The listing builds one solid part. Answer for the finished solid, in the listing's coordinates (mm). A direction names the side the tool comes from. Round coordinates to 2 decimals unless told otherwise and drop trailing zeros. Write each loop counter-clockwise with the first axis right and the second up, starting at its lowest first coordinate (ties: lowest second). Pieces come first, ordered by that corner, then holes.
Item 1: Find section A-A on z = 23. Give the vertices of the cut face in (x, y), then the cut area to 4 significant figures.
Item 2: Find section D-D on z = 9. Give the number of separate pieces and of enclosed holes in the cut face, then the cut area to 3 significant figures.
Item 3: For a pull along Y with two mould halves and no side action, classify faces 3 (the face through (-1, 34.5, 20)), 4 (the face through (-40.337, -31.317, 20.28)), 5 (the face through (-33.61, -21.49, 7.53)), 6 (the face through (-44.5, 0, 20)) as +Y half, -Y half, draft (parallel to the pull), parting line (faces both ways), or undercut.
Item 4: Each of these flat-tipped pins is pushed along its axis until it touches: pin 1 (18 mm diameter, centred on x = -4.5, y = 6.5, fed in from +Z); pin 2 (1.8 mm diameter, centred on x = -33.5, y = -21, fed in from +Z). Where does it stop, or does it pass through?
Item 5: Find section C-C on y = -22.5. Give the vertices of the cut face in (x, z).
Item 6: Find the intervals of material crossed by probe 1 along X at (y, z) = (-3, 37); probe 2 along Y at (x, z) = (15, 19.5); probe 3 along Y at (x, z) = (-32.5, 6.2), in increasing order.
Item 7: Find section B-B on x = 19.5. Give the vertices of the cut face in (y, z), then the cut area to 3 significant figures.
Item 8: A tool of negligible diameter and unlimited length cuts with its end or side. For faces 1 (the face through (-1, -30, 23)), 2 (the face through (0, -31, 40)), from which of +Z, -Z, +X, -X, +Y, -Y can it reach the whole face along a straight path? Write none if from no direction.
```python
from build123d import *

# Parameters (mm, degrees)
SKETCH_W        = 89
SKETCH_H        = 69
PAD_DEPTH       = 40
SKETCH001_W     = 80
SKETCH001_H     = 60
SKETCH001_R     = 3
SKETCH001_R_2   = 1.5
POCKET_DEPTH    = 35
SKETCH002_R     = 1.5
POCKET001_DEPTH = 40.001
SKETCH003_W     = 76.892074
SKETCH003_H     = 56.42009
POCKET002_DEPTH = 30
FILLET_R        = 3


with BuildPart() as part:
    # Sketch → Pad (new body)
    with BuildSketch(Plane.XY):
        Rectangle(SKETCH_W, SKETCH_H)
    extrude(amount=PAD_DEPTH)

    # Sketch001 (on DatumPlane) → Pocket (cut)
    with BuildSketch(Plane.XY.offset(40)):
        Rectangle(SKETCH001_W, SKETCH001_H)
        with Locations((-32.5, 22.5)):
            Circle(SKETCH001_R, mode=Mode.SUBTRACT)
        with Locations((32.5, 22.5)):
            Circle(SKETCH001_R, mode=Mode.SUBTRACT)
        with Locations((32.5, -22.5)):
            Circle(SKETCH001_R, mode=Mode.SUBTRACT)
        with Locations((-32.5, -22.5)):
            Circle(SKETCH001_R, mode=Mode.SUBTRACT)
        with Locations((-32.5, 22.5)):
            Circle(SKETCH001_R_2)
        with Locations((32.5, 22.5)):
            Circle(SKETCH001_R_2)
        with Locations((32.5, -22.5)):
            Circle(SKETCH001_R_2)
        with Locations((-32.5, -22.5)):
            Circle(SKETCH001_R_2)
    extrude(amount=-POCKET_DEPTH, mode=Mode.SUBTRACT)

    # Sketch002 (on DatumPlane) → Pocket001 (cut, through all)
    with BuildSketch(Plane.XY.offset(40)):
        with Locations((41.767767, 31.767767)):
            Circle(SKETCH002_R)
        with Locations((41.767767, -31.767767)):
            Circle(SKETCH002_R)
        with Locations((-41.767767, -31.767767)):
            Circle(SKETCH002_R)
        with Locations((-41.767767, 31.767767)):
            Circle(SKETCH002_R)
    extrude(amount=-POCKET001_DEPTH, mode=Mode.SUBTRACT)

    # Sketch003 (on DatumPlane) → Pocket002 (cut)
    with BuildSketch(Plane.XY.offset(40)):
        Rectangle(SKETCH003_W, SKETCH003_H)
    extrude(amount=-POCKET002_DEPTH, mode=Mode.SUBTRACT)

    # Fillet
    fillet_edges = [part.edges().sort_by_distance(p)[0] for p in [
        (-44.5, -34.5, 20),
        (44.5, -34.5, 20),
        (44.5, 34.5, 20),
        (-44.5, 34.5, 20),
    ]]
    fillet(fillet_edges, radius=FILLET_R)


solid = part.part
```
Check values:
1. outline: (-44.5, -31.5) arc R3 ccw to (-41.5, -34.5) - (41.5, -34.5) arc R3 ccw to (44.5, -31.5) - (44.5, 31.5) arc R3 ccw to (41.5, 34.5) - (-41.5, 34.5) arc R3 ccw to (-44.5, 31.5) - close; hole circle Ø3 at (-41.77, -31.77); hole circle Ø3 at (-41.77, 31.77); hole (-40, -30) - (40, -30) - (40, 30) - (-40, 30) - close; hole circle Ø3 at (41.77, -31.77); hole circle Ø3 at (41.77, 31.77)
1. area: 1,305 mm2
2. separate pieces: 5
2. enclosed holes: 9
2. area: 1,390 mm2
3. face 3: +Y half
3. face 4: undercut
3. face 5: undercut
3. face 6: draft
4. pin 1: stops at z = 5
4. pin 2: stops at z = 10
5. outline: (-44.5, 0) - (44.5, 0) - (44.5, 40) - (40, 40) - (40, 5) - (35.5, 5) - (35.5, 10) - (34, 10) - (34, 5) - (31, 5) - (31, 10) - (29.5, 10) - (29.5, 5) - (-29.5, 5) - (-29.5, 10) - (-31, 10) - (-31, 5) - (-34, 5) - (-34, 10) - (-35.5, 10) - (-35.5, 5) - (-40, 5) - (-40, 40) - (-44.5, 40) - close
6. probe 1: x = -44.5 to -40, 40 to 44.5
6. probe 2: y = -34.5 to -30, 30 to 34.5
6. probe 3: y = -34.5 to -30, -25.5 to -24, -21 to -19.5, 19.5 to 21, 24 to 25.5, 30 to 34.5
7. outline: (-34.5, 0) - (34.5, 0) - (34.5, 40) - (30, 40) - (30, 5) - (-30, 5) - (-30, 40) - (-34.5, 40) - close
7. area: 660 mm2
8. face 1: +Z
8. face 2: +Z, +X, -X, +Y, -Y
